```python
from build123d import *

# Parameters (mm, degrees)
SKETCH1_W               = 15
SKETCH1_H               = 10
BOSS_EXTRUDE1_DEPTH     = 35
FILLET1_R               = 7.5
CUT_EXTRUDE1_DEPTH      = 38.165171868
CUT_EXTRUDE1_DEPTH_BACK = 38.165171868
SKETCH2_R               = 2
FILLET2_R               = 1


with BuildPart() as part:
    # Sketch1 → Boss-Extrude1 (new body)
    with BuildSketch(Plane.XY):
        Rectangle(SKETCH1_W, SKETCH1_H)
    extrude(amount=BOSS_EXTRUDE1_DEPTH)

    # Fillet1
    fillet1_edges = [part.edges().sort_by_distance(p)[0] for p in [
        (7.5, 0, 35),
        (-7.5, 0, 35),
    ]]
    fillet(fillet1_edges, radius=FILLET1_R - 0.0001)  # a hair under: the kernel refuses the full size

    # Sketch2 → Cut-Extrude1 (cut, two sides: drawn at the far end of the back side and taken through both)
    with BuildSketch(Plane(origin=(0, 5, 0), x_dir=(1, 0, 0), z_dir=(0, 1, 0)).offset(-CUT_EXTRUDE1_DEPTH_BACK)):
        with Locations(Location((0, -27.5, 0), (0, 0, 180))):
            Circle(SKETCH2_R)
    extrude(amount=CUT_EXTRUDE1_DEPTH + CUT_EXTRUDE1_DEPTH_BACK, mode=Mode.SUBTRACT)

    # Fillet2
    fillet2_edges = [part.edges().sort_by_distance(p)[0] for p in [
        (7.5, 5, 13.75005),
        (7.5, -5, 13.75005),
        (-7.5, -5, 13.75005),
        (-5.303330148, -5, 32.803330148),
        (5.303330148, -5, 32.803330148),
        (-7.5, 5, 13.75005),
        (-5.303330148, 5, 32.803330148),
        (5.303330148, 5, 32.803330148),
        (2, -5, 27.5),
        (2, 5, 27.5),
    ]]
    fillet(fillet2_edges, radius=FILLET2_R)


solid = part.part
```
Design review of the part built by this model. Coordinates are the model's own, in mm. Give positions to 0.01 mm unless a question says otherwise; leave off trailing zeros.
(1) Clearance check with flat-ended pins moving along their axes: pin 1 Ø5 at (x, y) = (-3.5, 3) entering from +Z; pin 2 Ø3 at (x, z) = (0, 27.5) entering from +Y. State where each tip first meets the part, or that it passes through.
Checked values:
pin 1: stops at z = 34.93
pin 2: passes through
(2) Mouldability with a two-part tool opening along Z and no side actions: class faces 1 (the face through (0.434, -0.056, 25.548)), 2 (the face through (0, 0, 0)), 3 (the face through (5.361, 0.056, 32.745)), 4 (the face through (0, 5, 17)) as +Z half, -Z half, draft (parallel to the pull), parting line (faces both ways), or undercut.
Checked values:
face 1: undercut
face 2: -Z half
face 3: +Z half
face 4: draft
(3) Wall thickness on line 1 along Z through (x, y) = (0, -1.25); line 2 along X through (y, z) = (0, 27.5); line 3 along Z through (x, y) = (1.5, -4): over which ranges is each line inside the solid? List them lowest first.
Checked values:
line 1: z = 0 to 25.5, 29.5 to 35
line 2: x = -7.5 to -2, 2 to 7.5
line 3: z = 0 to 26.18, 28.82 to 34.85
